from build123d import *

# Parameters (mm, degrees)
SKETCH_1_W          = 140
SKETCH_1_H          = 100
EXTRUDE_1_DEPTH     = 3
SKETCH_2_R          = 13.25
SKETCH_2_R_2        = 2.15
CUT_EXTRUDE_1_DEPTH = 3
CUT_EXTRUDE_2_REACH = 88.076
SKETCH_4_R          = 1.75
SKETCH_4_R_2        = 1.65
EXTRUDE_2_DEPTH     = 3
FILLET_1_R          = 4
FILLET_2_R          = 3
CUT_EXTRUDE_3_REACH = 88.076
SKETCH_6_R          = 1.75


with BuildPart() as part:
    # Sketch 1 → Extrude 1 (new body)
    with BuildSketch(Plane(origin=(0, 0, 0), x_dir=(1, 0, 0), z_dir=(0, 1, 0))):
        Rectangle(SKETCH_1_W, SKETCH_1_H)
    extrude(amount=EXTRUDE_1_DEPTH)

    # Sketch 2 → Cut-Extrude 1 (cut)
    with BuildSketch(Plane(origin=(0, 3, 0), x_dir=(1, 0, 0), z_dir=(0, 1, 0))):
        with Locations(Location((0, -9, 0), (0, 0, 270))):
            Circle(SKETCH_2_R)
        with Locations(Location((12.347550503, -21.401128843, 0), (0, 0, 270))):
            Circle(SKETCH_2_R_2)
        with Locations(Location((12.401128843, 3.347550503, 0), (0, 0, 270))):
            Circle(SKETCH_2_R_2)
        with Locations(Location((-12.347550503, 3.401128843, 0), (0, 0, 270))):
            Circle(SKETCH_2_R_2)
        with Locations(Location((-12.401128843, -21.347550503, 0), (0, 0, 270))):
            Circle(SKETCH_2_R_2)
    extrude(amount=-CUT_EXTRUDE_1_DEPTH, mode=Mode.SUBTRACT)

    # Sketch 4 → Cut-Extrude 2 (cut, up to next)
    with BuildSketch(Plane(origin=(0, 3, 0), x_dir=(1, 0, 0), z_dir=(0, 1, 0)), mode=Mode.PRIVATE) as cut_extrude_2_sk1:
        with Locations(Location((-60, 40, 0), (0, 0, 270))):
            Circle(SKETCH_4_R)
    cut_extrude_2_tool1 = extrude(cut_extrude_2_sk1.sketch, amount=-CUT_EXTRUDE_2_REACH, mode=Mode.PRIVATE) & part.part
    # Sketch 4 → Cut-Extrude 2 (cut, up to next)
    with BuildSketch(Plane(origin=(0, 3, 0), x_dir=(1, 0, 0), z_dir=(0, 1, 0)), mode=Mode.PRIVATE) as cut_extrude_2_sk2:
        with Locations(Location((-60, -40, 0), (0, 0, 270))):
            Circle(SKETCH_4_R_2)
    cut_extrude_2_tool2 = extrude(cut_extrude_2_sk2.sketch, amount=-CUT_EXTRUDE_2_REACH, mode=Mode.PRIVATE) & part.part
    # Sketch 4 → Cut-Extrude 2 (cut, up to next)
    with BuildSketch(Plane(origin=(0, 3, 0), x_dir=(1, 0, 0), z_dir=(0, 1, 0)), mode=Mode.PRIVATE) as cut_extrude_2_sk3:
        with Locations(Location((60, -40, 0), (0, 0, 270))):
            Circle(SKETCH_4_R_2)
    cut_extrude_2_tool3 = extrude(cut_extrude_2_sk3.sketch, amount=-CUT_EXTRUDE_2_REACH, mode=Mode.PRIVATE) & part.part
    # Sketch 4 → Cut-Extrude 2 (cut, up to next)
    with BuildSketch(Plane(origin=(0, 3, 0), x_dir=(1, 0, 0), z_dir=(0, 1, 0)), mode=Mode.PRIVATE) as cut_extrude_2_sk4:
        with Locations(Location((60, 40, 0), (0, 0, 270))):
            Circle(SKETCH_4_R)
    cut_extrude_2_tool4 = extrude(cut_extrude_2_sk4.sketch, amount=-CUT_EXTRUDE_2_REACH, mode=Mode.PRIVATE) & part.part
    # Sketch 4 → Cut-Extrude 2 (cut, up to next)
    with BuildSketch(Plane(origin=(0, 3, 0), x_dir=(1, 0, 0), z_dir=(0, 1, 0)), mode=Mode.PRIVATE) as cut_extrude_2_sk5:
        with BuildLine():
            Line((13.564659966, -30), (50, -30))
            Line((50, -30), (50, 30))
            Line((50, 30), (-50, 30))
            Line((-50, 30), (-50, -30))
            Line((-50, -30), (-13.564659966, -30))
            ThreePointArc((-13.564659966, -30), (0, 16), (13.564659966, -30))
        make_face()
    cut_extrude_2_tool5 = extrude(cut_extrude_2_sk5.sketch, amount=-CUT_EXTRUDE_2_REACH, mode=Mode.PRIVATE) & part.part
    add(cut_extrude_2_tool1.solids().sort_by_distance((-60, 3, -40))[0], mode=Mode.SUBTRACT)
    add(cut_extrude_2_tool2.solids().sort_by_distance((-60, 3, 40))[0], mode=Mode.SUBTRACT)
    add(cut_extrude_2_tool3.solids().sort_by_distance((60, 3, 40))[0], mode=Mode.SUBTRACT)
    add(cut_extrude_2_tool4.solids().sort_by_distance((60, 3, -40))[0], mode=Mode.SUBTRACT)
    add(cut_extrude_2_tool5.solids().sort_by_distance((31.78233, 3, 28.83381))[0], mode=Mode.SUBTRACT)

    # Sketch 5 → Extrude 2 (add)
    with BuildSketch(Plane(origin=(0, 3, 0), x_dir=(1, 0, 0), z_dir=(0, 1, 0))):
        Polygon((46.998056898, 33.999619926), (12.318341703, 6.949442073), (18.46865969, -0.935580987), (53.001943102, 26.000380074), align=None)
        Polygon((-18.46865969, -0.935580987), (-53.001943102, 26.000380074), (-46.998056898, 33.999619926), (-12.318341703, 6.949442073), align=None)
    extrude(amount=-EXTRUDE_2_DEPTH)

    # Fillet 1
    fillet_1_edges = [part.edges().sort_by_distance(p)[0] for p in [
        (50, 1.5, -23.658864455),
        (16.239124114, 1.5, -10.007652354),
        (-22.389442101, 1.5, -2.122629294),
        (-16.239124114, 1.5, -10.007652354),
        (50, 1.5, 30),
        (13.564659966, 1.5, 30),
        (-13.564659966, 1.5, 30),
        (-50, 1.5, 30),
        (-41.870339045, 1.5, -30),
        (41.870339045, 1.5, -30),
        (-50, 1.5, -23.658864455),
        (22.389442101, 1.5, -2.122629294),
    ]]
    fillet(fillet_1_edges, radius=FILLET_1_R)

    # Fillet 2
    fillet_2_edges = [part.edges().sort_by_distance(p)[0] for p in [
        (70, 1.5, 50),
        (-70, 1.5, 50),
        (-70, 1.5, -50),
        (70, 1.5, -50),
    ]]
    fillet(fillet_2_edges, radius=FILLET_2_R)

    # Sketch 6 → Cut-Extrude 3 (cut, up to next)
    with BuildSketch(Plane(origin=(0, 3, 0), x_dir=(1, 0, 0), z_dir=(0, 1, 0)), mode=Mode.PRIVATE) as cut_extrude_3_sk1:
        with Locations(Location((-40, 40, 0), (0, 0, 270))):
            Circle(SKETCH_6_R)
    cut_extrude_3_tool1 = extrude(cut_extrude_3_sk1.sketch, amount=-CUT_EXTRUDE_3_REACH, mode=Mode.PRIVATE) & part.part
    # Sketch 6 → Cut-Extrude 3 (cut, up to next)
    with BuildSketch(Plane(origin=(0, 3, 0), x_dir=(1, 0, 0), z_dir=(0, 1, 0)), mode=Mode.PRIVATE) as cut_extrude_3_sk2:
        with Locations(Location((-20, 40, 0), (0, 0, 270))):
            Circle(SKETCH_6_R)
    cut_extrude_3_tool2 = extrude(cut_extrude_3_sk2.sketch, amount=-CUT_EXTRUDE_3_REACH, mode=Mode.PRIVATE) & part.part
    # Sketch 6 → Cut-Extrude 3 (cut, up to next)
    with BuildSketch(Plane(origin=(0, 3, 0), x_dir=(1, 0, 0), z_dir=(0, 1, 0)), mode=Mode.PRIVATE) as cut_extrude_3_sk3:
        with Locations(Location((-60, 20, 0), (0, 0, 270))):
            Circle(SKETCH_6_R)
    cut_extrude_3_tool3 = extrude(cut_extrude_3_sk3.sketch, amount=-CUT_EXTRUDE_3_REACH, mode=Mode.PRIVATE) & part.part
    # Sketch 6 → Cut-Extrude 3 (cut, up to next)
    with BuildSketch(Plane(origin=(0, 3, 0), x_dir=(1, 0, 0), z_dir=(0, 1, 0)), mode=Mode.PRIVATE) as cut_extrude_3_sk4:
        with Locations(Location((-60, -20, 0), (0, 0, 270))):
            Circle(SKETCH_6_R)
    cut_extrude_3_tool4 = extrude(cut_extrude_3_sk4.sketch, amount=-CUT_EXTRUDE_3_REACH, mode=Mode.PRIVATE) & part.part
    # Sketch 6 → Cut-Extrude 3 (cut, up to next)
    with BuildSketch(Plane(origin=(0, 3, 0), x_dir=(1, 0, 0), z_dir=(0, 1, 0)), mode=Mode.PRIVATE) as cut_extrude_3_sk5:
        with Locations(Location((-60, 0, 0), (0, 0, 270))):
            Circle(SKETCH_6_R)
    cut_extrude_3_tool5 = extrude(cut_extrude_3_sk5.sketch, amount=-CUT_EXTRUDE_3_REACH, mode=Mode.PRIVATE) & part.part
    # Sketch 6 → Cut-Extrude 3 (cut, up to next)
    with BuildSketch(Plane(origin=(0, 3, 0), x_dir=(1, 0, 0), z_dir=(0, 1, 0)), mode=Mode.PRIVATE) as cut_extrude_3_sk6:
        with Locations(Location((-40, -40, 0), (0, 0, 270))):
            Circle(SKETCH_6_R)
    cut_extrude_3_tool6 = extrude(cut_extrude_3_sk6.sketch, amount=-CUT_EXTRUDE_3_REACH, mode=Mode.PRIVATE) & part.part
    add(cut_extrude_3_tool1.solids().sort_by_distance((-40, 3, -40))[0], mode=Mode.SUBTRACT)
    add(cut_extrude_3_tool2.solids().sort_by_distance((-20, 3, -40))[0], mode=Mode.SUBTRACT)
    add(cut_extrude_3_tool3.solids().sort_by_distance((-60, 3, -20))[0], mode=Mode.SUBTRACT)
    add(cut_extrude_3_tool4.solids().sort_by_distance((-60, 3, 20))[0], mode=Mode.SUBTRACT)
    add(cut_extrude_3_tool5.solids().sort_by_distance((-60, 3, 0))[0], mode=Mode.SUBTRACT)
    add(cut_extrude_3_tool6.solids().sort_by_distance((-40, 3, 40))[0], mode=Mode.SUBTRACT)


solid = part.part
Model file for the job. Use its own axes, mm. Give positions to 0.01 mm unless a question says otherwise; leave off trailing zeros. Order: outer loops, then holes, each group sorted by start corner. A loop starts at its lowest first (then second) coordinate and runs counter-clockwise, first axis right, second up. Notation, with made-up numbers: M 49.5,58 L 58.5,58 A18 ccw 58.5,83 Z; hole C 60.5,-36 d10. An arc over 180 degrees is marked long. Write item = value, one per line.
Q1. Cut at A-A, the plane x = 0. List the corners of the cut face in (y, z), then the cut area to 4 significant figures.
Derived:
outline = M 0,-50 L 3,-50 L 3,-30 L 0,-30 Z; M 0,-16 L 3,-16 L 3,-4.25 L 0,-4.25 Z; M 0,22.25 L 3,22.25 L 3,50 L 0,50 Z
area = 178.5 mm2
Q2. Cut at B-B, the plane z = 40. List the corners of the cut face in (x, y).
Derived:
outline = M -70,0 L -61.65,0 L -61.65,3 L -70,3 Z; M -58.35,0 L -41.75,0 L -41.75,3 L -58.35,3 Z; M -38.25,0 L 58.35,0 L 58.35,3 L -38.25,3 Z; M 61.65,0 L 70,0 L 70,3 L 61.65,3 Z
Q3. Cut at C-C, the plane x = -60. List the corners of the cut face in (y, z).
Derived:
outline = M 0,-50 L 3,-50 L 3,-41.75 L 0,-41.75 Z; M 0,-38.25 L 3,-38.25 L 3,-21.75 L 0,-21.75 Z; M 0,-18.25 L 3,-18.25 L 3,-1.75 L 0,-1.75 Z; M 0,1.75 L 3,1.75 L 3,18.25 L 0,18.25 Z; M 0,21.75 L 3,21.75 L 3,38.35 L 0,38.35 Z; M 0,41.65 L 3,41.65 L 3,50 L 0,50 Z
Q4. Two-plate mould, pull along Z, no slides. Class faces 1 (the cylindrical face through (-61.71, 1.52, -0.38)), 2 (the flat face through (-1, 3, -12)), 3 (the flat face through (-1, 1, -50)): pulls with the +Z half, pulls with the -Z half, needs draft (parallel to the pull), parting line crosses it, or undercut.
Derived:
face_1 = undercut
face_2 = needs draft
face_3 = pulls with the -Z half
Q5. Cut at D-D, the plane z = -40. List the corners of the cut face in (x, y), then the cut area to 3 significant figures.
Derived:
outline = M -70,0 L -61.75,0 L -61.75,3 L -70,3 Z; M -58.25,0 L -41.75,0 L -41.75,3 L -58.25,3 Z; M -38.25,0 L -21.75,0 L -21.75,3 L -38.25,3 Z; M -18.25,0 L 58.25,0 L 58.25,3 L -18.25,3 Z; M 61.75,0 L 70,0 L 70,3 L 61.75,3 Z
area = 378 mm2
Q6. Drill centre lines: line 1 (X direction, y = 2.45, z = 0.5); line 2 (X direction, y = 2.1, z = -40); line 3 (X direction, y = 1.8, z = 39.5). Where is each one in solid material? Low to high. Write a range as [from, to].
Derived:
line_1 = [-70, -61.68], [-58.32, -50], [-23.51, -10.16], [10.16, 23.51], [50, 70]
line_2 = [-70, -61.75], [-58.25, -41.75], [-38.25, -21.75], [-18.25, 58.25], [61.75, 70]
line_3 = [-70, -61.57], [-58.43, -41.68], [-38.32, 58.43], [61.57, 70]
